Design review of the part built by this model. Coordinates are the model's own, in mm. Face numbers are marked on the shaded views. A direction names the side the tool comes from. Coordinates: 2 decimals unless noted, no trailing zeros. Loops run counter-clockwise (first coordinate to the right, second up) from the corner with the lowest first, then second, coordinate; pieces in that order, holes last. Notation, with made-up numbers: M 34,-29.75 L 57,-29.75 A18 cw 57,-0.75 Z; hole C 75,74.25 d1. An arc over 180 degrees is marked long. Answer as a JSON object with one key per item and string values. Group by question number.
1. To check wall thickness, follow probe 1 along Z at (x, y) = (7.5, 45.75); probe 2 along Y at (x, z) = (10, 0); probe 3 along Y at (x, z) = (6, 0). State the ranges of each line that lie inside material, in increasing order.
2. Consider section B-B (z = 0). State the section outline as (x, y) points.
3. Consider section A-A (y = 50.4). State the section outline as (x, z) points, then the cut area to 3 significant figures.
4. Consider section C-C (x = 21.5). State the section outline as (y, z) points, then the cut area to 3 significant figures.
5. Machinability: for the marked faces 4 and 5, which of the approach directions +Z, -Z, +X, -X, +Y, -Y give a long, thin tool a straight path to every point of the face, cutting with its end or side? Answer none if there is none.
6. Insertion check: pin 1 (8 mm diameter, centred on x = 14.5, z = 0, fed in from +Y); pin 2 (2 mm diameter, centred on y = 46.5, z = -12, fed in from +X). Each pin has a flat end and moves straight along its axis. Give the tip position at first contact, or say it passes through.
7. Draft analysis for pull direction X (two halves, no side actions). For the marked faces 1, 2 and 3, state which applies: +X half, -X half, draft (parallel to the pull), parting line (faces both ways), or undercut.
8. Consider section D-D (y = 45.75). State the section outline as (x, z) points, then the cut area to 3 significant figures.
from build123d import *

# Parameters (mm, degrees)
SKETCH1_W           = 65
SKETCH1_H           = 30
BOSS_EXTRUDE1_DEPTH = 58
FILLET1_R           = 13
SKETCH15_W          = 83.696095513
SKETCH15_H          = 31.69844841
CUT_EXTRUDE7_DEPTH  = 50
SKETCH18_R          = 16
CUT_EXTRUDE10_DEPTH = 5.5
SKETCH3_R           = 1.6
CUT_EXTRUDE12_DEPTH = 89.396832522
SKETCH21_W          = 2
SKETCH21_H          = 2
CUT_EXTRUDE13_DEPTH = 8


with BuildPart() as part:
    # Sketch1 → Boss-Extrude1 (new body)
    with BuildSketch(Plane(origin=(0, 0, 0), x_dir=(1, 0, 0), z_dir=(0, 1, 0))):
        with Locations((7.5, 0)):
            Rectangle(SKETCH1_W, SKETCH1_H)
    extrude(amount=BOSS_EXTRUDE1_DEPTH)

    # Fillet1
    fillet1_edges = [part.edges().sort_by_distance(p)[0] for p in [
        (40, 29, 15),
        (-25, 29, 15),
        (-25, 29, -15),
        (40, 29, -15),
    ]]
    fillet(fillet1_edges, radius=FILLET1_R)

    # Sketch15 → Cut-Extrude7 (cut)
    with BuildSketch(Plane(origin=(0, -10, 0), x_dir=(-1, 0, 0), z_dir=(0, -1, 0))):
        with Locations((-0.057440767, 0.030479277)):
            Rectangle(SKETCH15_W, SKETCH15_H)
    extrude(amount=-CUT_EXTRUDE7_DEPTH, mode=Mode.SUBTRACT)

    # Sketch18 → Cut-Extrude10 (cut)
    with BuildSketch(Plane(origin=(0, 58, 0), x_dir=(1, 0, 0), z_dir=(0, 1, 0))):
        with Locations((6.828508286, 0)):
            Circle(SKETCH18_R)
    extrude(amount=-CUT_EXTRUDE10_DEPTH, mode=Mode.SUBTRACT)

    # Sketch3 → Cut-Extrude12 (cut, through all)
    with BuildSketch(Plane.ZY.offset(25)):
        with Locations((0, 50.4)):
            Circle(SKETCH3_R)
    extrude(amount=-CUT_EXTRUDE12_DEPTH, mode=Mode.SUBTRACT)

    # Sketch21 → Cut-Extrude13 (cut)
    with BuildSketch(Plane(origin=(0, 52.5, 0), x_dir=(1, 0, 0), z_dir=(0, 1, 0))):
        with Locations((6.828508286, 0)):
            Rectangle(SKETCH21_W, SKETCH21_H)
    extrude(amount=-CUT_EXTRUDE13_DEPTH, mode=Mode.SUBTRACT)


solid = part.part
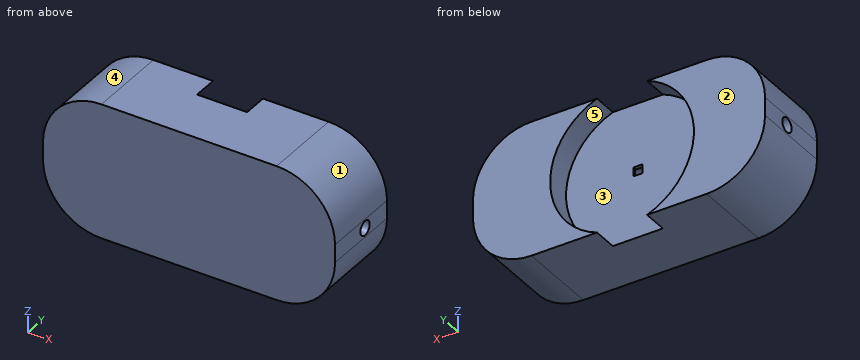
Findings below:
{
 "1": {"probe 1": "z = -15 to -1, 1 to 15", "probe 2": "y = 40 to 48.8, 52 to 52.5", "probe 3": "y = 40 to 44.5"},
 "2": {"outline": "M -25,40 L 40,40 L 40,48.8 L 7.83,48.8 L 7.83,44.5 L 5.83,44.5 L 5.83,48.8 L -25,48.8 Z; M -25,52 L 5.83,52 L 5.83,52.5 L -9.17,52.5 L -9.17,58 L -25,58 Z; M 7.83,52 L 40,52 L 40,58 L 22.83,58 L 22.83,52.5 L 7.83,52.5 Z"},
 "3": {"outline": "M -25,-2 A13 ccw -12,-15 L 27,-15 A13 ccw 40,-2 L 40,-1.6 L -25,-1.6 Z; M -25,1.6 L 40,1.6 L 40,2 A13 ccw 27,15 L -12,15 A13 ccw -25,2 Z", "area": "1,600 mm^2"},
 "4": {"outline": "M 40,-15 L 58,-15 L 58,-6.38 L 52.5,-6.38 L 52.5,6.38 L 58,6.38 L 58,15 L 40,15 Z; hole C 50.4,0 d3.2", "area": "462 mm^2"},
 "5": {"face 4": "+Z, -X, +Y, -Y", "face 5": "+Y"},
 "6": {"pin 1": "stops at y = 52.5", "pin 2": "stops at x = 36.38"},
 "7": {"face 1": "+X half", "face 2": "draft", "face 3": "undercut"},
 "8": {"outline": "M -25,-2 A13 ccw -12,-15 L 27,-15 A13 ccw 40,-2 L 40,2 A13 ccw 27,15 L -12,15 A13 ccw -25,2 Z; hole M 5.83,-1 L 7.83,-1 L 7.83,1 L 5.83,1 Z", "area": "1,800 mm^2"}
}
